```python
from build123d import *

# Parameters (mm, degrees)
SKETCH_1_W          = 20
SKETCH_1_H          = 40
SKETCH_1_W_2        = 17
SKETCH_1_H_2        = 37
EXTRUDE_1_DEPTH     = 250
SKETCH_2_R          = 2
CUT_EXTRUDE_1_DEPTH = 252.594912508
SKETCH_3_R          = 2.1
CUT_EXTRUDE_2_DEPTH = 254.377189186
SKETCH_4_R          = 1.6
CUT_EXTRUDE_3_DEPTH = 254.377189186
SKETCH_5_R          = 4
CUT_EXTRUDE_4_DEPTH = 10
SKETCH_6_R          = 4
CUT_EXTRUDE_5_DEPTH = 10


with BuildPart() as part:
    # 草图1 → 凸台-拉伸1 (new body)
    with BuildSketch(Plane.XY):
        Rectangle(SKETCH_1_W, SKETCH_1_H)
        Rectangle(SKETCH_1_W_2, SKETCH_1_H_2, mode=Mode.SUBTRACT)
    extrude(amount=-EXTRUDE_1_DEPTH)

    # 草图2 → 切除-拉伸1 (cut, through all)
    with BuildSketch(Plane.ZY.offset(10)):
        with Locations((-100, 6)):
            Circle(SKETCH_2_R)
        with Locations((-52, 6)):
            Circle(SKETCH_2_R)
        with Locations((-52, -6)):
            Circle(SKETCH_2_R)
        with Locations((-100, -6)):
            Circle(SKETCH_2_R)
        with Locations((-150, -6)):
            Circle(SKETCH_2_R)
        with Locations((-198, -6)):
            Circle(SKETCH_2_R)
        with Locations((-198, 6)):
            Circle(SKETCH_2_R)
        with Locations((-150, 6)):
            Circle(SKETCH_2_R)
    extrude(amount=-CUT_EXTRUDE_1_DEPTH, mode=Mode.SUBTRACT)

    # 草图3 → 切除-拉伸2 (cut, through all)
    with BuildSketch(Plane(origin=(0, 20, 0), x_dir=(1, 0, 0), z_dir=(0, 1, 0))):
        with Locations(Location((0, 22.5, 0), (0, 0, 270))):
            Circle(SKETCH_3_R)
        with Locations(Location((0, 7.5, 0), (0, 0, 270))):
            Circle(SKETCH_3_R)
        with Locations(Location((0, 242.5, 0), (0, 0, 270))):
            Circle(SKETCH_3_R)
        with Locations(Location((0, 227.5, 0), (0, 0, 270))):
            Circle(SKETCH_3_R)
    extrude(amount=-CUT_EXTRUDE_2_DEPTH, mode=Mode.SUBTRACT)

    # 草图4 → 切除-拉伸3 (cut, through all)
    with BuildSketch(Plane(origin=(0, 20, 0), x_dir=(1, 0, 0), z_dir=(0, 1, 0))):
        with Locations(Location((0, 130, 0), (0, 0, 270))):
            Circle(SKETCH_4_R)
        with Locations(Location((0, 120, 0), (0, 0, 270))):
            Circle(SKETCH_4_R)
    extrude(amount=-CUT_EXTRUDE_3_DEPTH, mode=Mode.SUBTRACT)

    # 草图5 → 切除-拉伸4 (cut)
    with BuildSketch(Plane(origin=(0, 20, 0), x_dir=(1, 0, 0), z_dir=(0, 1, 0))):
        with Locations(Location((0, 22.5, 0), (0, 0, 270))):
            Circle(SKETCH_5_R)
        with Locations(Location((0, 7.5, 0), (0, 0, 270))):
            Circle(SKETCH_5_R)
        with Locations(Location((0, 242.5, 0), (0, 0, 270))):
            Circle(SKETCH_5_R)
        with Locations(Location((0, 227.5, 0), (0, 0, 270))):
            Circle(SKETCH_5_R)
    extrude(amount=-CUT_EXTRUDE_4_DEPTH, mode=Mode.SUBTRACT)

    # 草图6 → 切除-拉伸5 (cut)
    with BuildSketch(Plane(origin=(10, 0, 0), x_dir=(0, 0, -1), z_dir=(1, 0, 0))):
        with Locations((52, 6)):
            Circle(SKETCH_6_R)
        with Locations((52, -6)):
            Circle(SKETCH_6_R)
        with Locations((198, 6)):
            Circle(SKETCH_6_R)
        with Locations((198, -6)):
            Circle(SKETCH_6_R)
    extrude(amount=-CUT_EXTRUDE_5_DEPTH, mode=Mode.SUBTRACT)


solid = part.part
```
Model file for the job. Use its own axes, mm. A direction names the side the tool comes from. Give positions to 0.01 mm unless a question says otherwise; leave off trailing zeros. Order: outer loops, then holes, each group sorted by start corner. A loop starts at its lowest first (then second) coordinate and runs counter-clockwise, first axis right, second up.
1) Saw through at B-B, the plane y = 14. Write the cut outline in (x, z).
2) Saw through at A-A, the plane z = -168. Write the cut outline in (x, y), then the cut area to 3 significant figures.
3) Wall check: probe 1 along Y at (x, z) = (9.35, -52); probe 2 along X at (y, z) = (15.5, -223); probe 3 along Y at (x, z) = (-0.75, -174). Give the ranges that are in metal, low to high.
4) 3-axis set-ups, long thin cutter, end or side, ignore diameter. For faces 1 (the flat face through (-8.5, 0, -123)), 2 (the cylindrical face through (-2.4, 19.3, -10.7)), 3 (the cylindrical face through (9.26, 7.201, -201.815)): which of +Z, -Z, +X, -X, +Y, -Y reach the whole face in a straight line?
5) Saw through at C-C, the plane z = -242.5. Write the cut outline in (x, y), then the cut area to 3 significant figures.
6) Pin check, flat tip, straight feed: pin 1 (2.5 mm diameter, centred on y = -6, z = -150, fed in from +X). Stop position of the tip, or through.
7) Mould opens along Y. For faces 4 (the cylindrical face through (-9, 6, -200)), 5 (the cylindrical face through (0.176, 19.26, -246.496)), 6 (the cylindrical face through (9.24, 6.601, -98.092)), 7 (the flat face through (0, -20, -123)) say: +Y half, -Y half, draft (parallel to the pull), parting line (faces both ways), or undercut.
Computed:
1. outline: (-10, -250) - (-8.5, -250) - (-8.5, 0) - (-10, 0) - close; (8.5, -250) - (10, -250) - (10, 0) - (8.5, 0) - close
2. outline: (-10, -20) - (10, -20) - (10, 20) - (-10, 20) - close; hole (-8.5, -18.5) - (8.5, -18.5) - (8.5, 18.5) - (-8.5, 18.5) - close
2. area: 171 mm2
3. probe 1: y = -20 to -10, -2 to 2, 10 to 20
3. probe 2: x = -10 to -8.5, 8.5 to 10
3. probe 3: y = -20 to -18.5, 18.5 to 20
4. face 1: +Z, -Z
4. face 2: +Y
4. face 3: +X
5. outline: (-10, -20) - (-2.1, -20) - (-2.1, -18.5) - (-8.5, -18.5) - (-8.5, 18.5) - (-4, 18.5) - (-4, 20) - (-10, 20) - close; (2.1, -20) - (10, -20) - (10, 20) - (4, 20) - (4, 18.5) - (8.5, 18.5) - (8.5, -18.5) - (2.1, -18.5) - close
5. area: 153 mm2
6. pin 1: passes through
7. face 4: undercut
7. face 5: draft
7. face 6: undercut
7. face 7: -Y half
